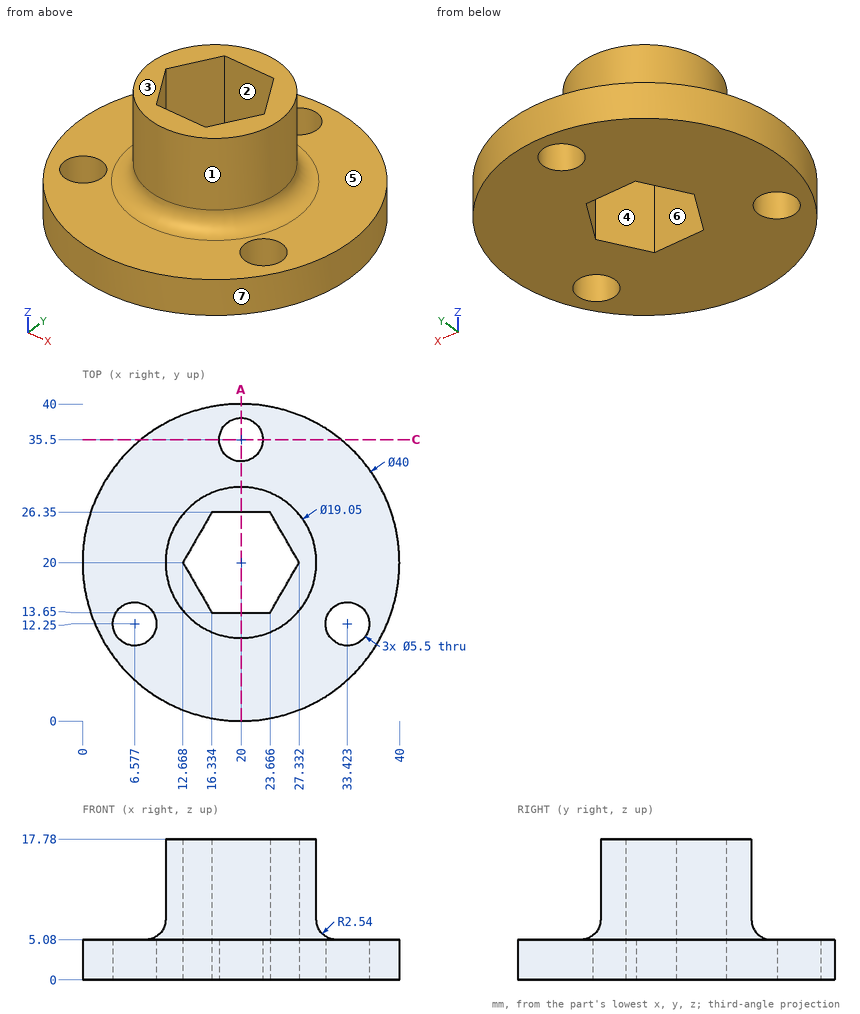
The figure shows three views and two pictorial views of one solid part (mm, origin at its lowest corner). Answer the questions. A direction names the side the tool comes from. Give positions to 0.01 mm unless a question says otherwise; leave off trailing zeros. Order: outer loops, then holes, each group sorted by start corner. A loop starts at its lowest first (then second) coordinate and runs counter-clockwise, first axis right, second up. Notation, with made-up numbers: (3.5, 17) -> (40.5, 17) arc R25 ccw to (40.5, 55) -> close; hole circle Ø1 at (-28, -39.5). An arc over 180 degrees is marked (long way). Answer as CSV lines item,"result". Start each with the question number.
(1) Which of the six approach directions +Z, -Z, +X, -X, +Y, -Y give full straight-line access (tool end or side, diameter ignored) to the marked faces 1, 2 and 3?
(2) Section A-A, the plane x = 20 is taken. Give the number of separate pieces and of enclosed holes in the cut face, plus the area to 3 significant figures.
(3) Consider line 1 along Y through (x, z) = (20, 1.35); line 2 along Z through (x, y) = (3, 14.5); line 3 along Y through (x, z) = (15, 4.75) (1 decimal). Determine where each line is inside the solid, lowest interval first.
(4) For a pull along X with two mould halves and no side action, classify the marked faces 4, 5, 6 and 7 as released by +X, released by -X, zero draft, split by the parting line, or undercut.
(5) Section C-C, the plane y = 35.5 is taken. Write down the section's boundary in (x, z).
(6) Each of these flat-tipped pins is pushed along its axis until it touches: pin 1 Ø10 at (y, z) = (11.5, 14) entering from +X; pin 2 Ø8 at (y, z) = (12, 4.5) entering from +X; pin 3 Ø4 at (y, z) = (20, 7) entering from +X; pin 4 Ø8 at (x, z) = (19, 13.5) entering from -Y (3 decimals). Where does it stop, or does it pass through?
Entries:
1,face 1,"+Z"
1,face 2,"+Z, -Z"
1,face 3,"+Z, +X, -X, +Y, -Y"
2,separate pieces,"3"
2,enclosed holes,"0"
2,area,"194 mm²"
3,line 1,"0 to 13.65, 26.35 to 32.75, 38.25 to 40"
3,line 2,"0 to 5.08"
3,line 3,"0.6 to 16, 24 to 39.4"
4,face 4,"undercut"
4,face 5,"zero draft"
4,face 6,"undercut"
4,face 7,"split by the parting line"
5,outline,"(7.36, 0) -> (17.25, 0) -> (17.25, 5.08) -> (7.36, 5.08) -> close; (22.75, 0) -> (32.64, 0) -> (32.64, 5.08) -> (22.75, 5.08) -> close"
6,pin 1,"x = 28.86"
6,pin 2,"x = 39.6"
6,pin 3,"x = 40"
6,pin 4,"y = 10.475"
